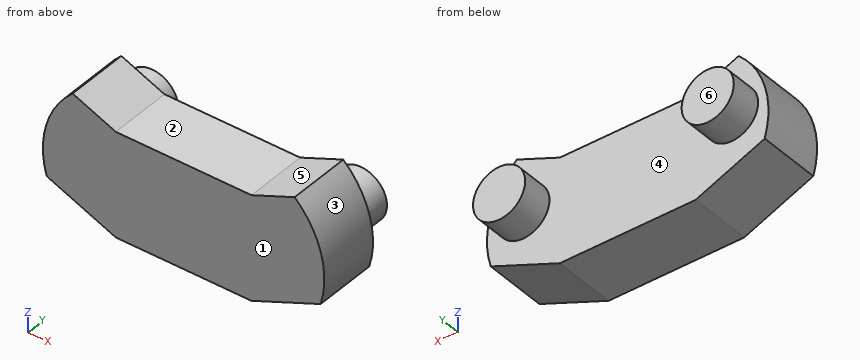
```python
from build123d import *

# Parameters (mm, degrees)
SKETCH2_W           = 32.5
SKETCH2_H           = 50
BOSS_EXTRUDE1_DEPTH = 30
FILLET1_R           = 3
SKETCH3_R           = 12.5
BOSS_EXTRUDE2_DEPTH = 45
CUT_EXTRUDE1_DEPTH  = 92.572762002


with BuildPart() as part:
    # Sketch2 → Boss-Extrude1 (new body)
    with BuildSketch(Plane(origin=(0, 0, 0), x_dir=(1, 0, 0), z_dir=(0, 1, 0))):
        with BuildLine():
            Line((-33.026431533, 15.07807147), (-21.486968519, 36.349341511))
            Line((-21.486968519, 36.349341511), (-56.486968519, 21.832088794))
            Line((-56.486968519, 21.832088794), (-47.76505884, 12.989879738))
            ThreePointArc((-47.76505884, 12.989879738), (-40.740475826, 16.467112533), (-33.026431533, 15.07807147))
        make_face()
        with BuildLine():
            Line((-47.76505884, 12.989879738), (-56.486968519, 21.832088794))
            Line((-56.486968519, 21.832088794), (-56.486968519, -28.167911206))
            Line((-56.486968519, -28.167911206), (-44.947505506, -6.896641164))
            ThreePointArc((-44.947505506, -6.896641164), (-51.3633659, 2.337207846), (-47.76505884, 12.989879738))
        make_face()
        with BuildLine():
            Line((-56.486968519, -28.167911206), (-21.486968519, -13.650658489))
            Line((-21.486968519, -13.650658489), (-30.208878198, -4.808449432))
            ThreePointArc((-30.208878198, -4.808449432), (-37.233461212, -8.285682228), (-44.947505506, -6.896641164))
            Line((-44.947505506, -6.896641164), (-56.486968519, -28.167911206))
        make_face()
        with BuildLine():
            Line((-21.486968519, -13.650658489), (-21.486968519, 36.349341511))
            Line((-21.486968519, 36.349341511), (-33.026431533, 15.07807147))
            ThreePointArc((-33.026431533, 15.07807147), (-28.245536763, 10.483808601), (-26.486968519, 4.090715153))
            ThreePointArc((-26.486968519, 4.090715153), (-27.454923405, -0.732347722), (-30.208878198, -4.808449432))
            Line((-30.208878198, -4.808449432), (-21.486968519, -13.650658489))
        make_face()
        with Locations((-5.236968519, 11.349341511)):
            Rectangle(SKETCH2_W, SKETCH2_H)
        with BuildLine():
            Line((55.052494494, 15.07807147), (43.513031481, 36.349341511))
            Line((43.513031481, 36.349341511), (43.513031481, -13.650658489))
            Line((43.513031481, -13.650658489), (52.23494116, -4.808449432))
            ThreePointArc((52.23494116, -4.808449432), (48.6366341, 5.84422246), (55.052494494, 15.07807147))
        make_face()
        with BuildLine():
            Line((78.513031481, 21.832088794), (43.513031481, 36.349341511))
            Line((43.513031481, 36.349341511), (55.052494494, 15.07807147))
            ThreePointArc((55.052494494, 15.07807147), (62.766538788, 16.467112533), (69.791121802, 12.989879738))
            Line((69.791121802, 12.989879738), (78.513031481, 21.832088794))
        make_face()
        with BuildLine():
            Line((78.513031481, -28.167911206), (78.513031481, 21.832088794))
            Line((78.513031481, 21.832088794), (69.791121802, 12.989879738))
            ThreePointArc((69.791121802, 12.989879738), (72.545076595, 8.913778028), (73.513031481, 4.090715153))
            ThreePointArc((73.513031481, 4.090715153), (71.754463237, -2.302378295), (66.973568467, -6.896641164))
            Line((66.973568467, -6.896641164), (78.513031481, -28.167911206))
        make_face()
        with BuildLine():
            Line((52.23494116, -4.808449432), (43.513031481, -13.650658489))
            Line((43.513031481, -13.650658489), (78.513031481, -28.167911206))
            Line((78.513031481, -28.167911206), (66.973568467, -6.896641164))
            ThreePointArc((66.973568467, -6.896641164), (59.259524174, -8.285682228), (52.23494116, -4.808449432))
        make_face()
        with Locations((27.263031481, 11.349341511)):
            Rectangle(SKETCH2_W, SKETCH2_H)
    extrude(amount=BOSS_EXTRUDE1_DEPTH)

    # Fillet1
    fillet1_edges = [part.edges().sort_by_distance(p)[0] for p in [
        (-56.486968519, 15, 28.167911206),
        (-56.486968519, 15, -21.832088794),
        (78.513031481, 15, -21.832088794),
        (78.513031481, 15, 28.167911206),
    ]]
    fillet(fillet1_edges, radius=FILLET1_R)

    # Sketch3 → Boss-Extrude2 (add)
    with BuildSketch(Plane(origin=(0, 0, 0), x_dir=(-1, 0, 0), z_dir=(0, -1, 0))):
        with Locations(Location((38.986968519, 4.090715153, 0), (0, 0, 90))):
            Circle(SKETCH3_R)
        with Locations(Location((-61.013031481, 4.090715153, 0), (0, 0, 90))):
            Circle(SKETCH3_R)
    extrude(amount=-BOSS_EXTRUDE2_DEPTH)

    # Sketch4 → Cut-Extrude1 (cut, through all)
    with BuildSketch(Plane(origin=(0, 30, 0), x_dir=(1, 0, 0), z_dir=(0, 1, 0))):
        with BuildLine():
            ThreePointArc((-56.486968519, -23.675749532), (-55.153077724, -26.17056017), (-52.337581774, -26.446834177))
            Line((-52.337581774, -26.446834177), (-42.18410533, -22.235388934))
            ThreePointArc((-42.18410533, -22.235388934), (-54.833584995, -1.601840339), (-54.636355265, 22.59968366))
            ThreePointArc((-54.636355265, 22.59968366), (-55.981779157, 21.494708219), (-56.486968519, 19.828599015))
            Line((-56.486968519, 19.828599015), (-56.486968519, -23.675749532))
        make_face()
        with BuildLine():
            Line((64.210168291, -22.235388934), (74.363644735, -26.446834177))
            ThreePointArc((74.363644735, -26.446834177), (77.179140685, -26.17056017), (78.513031481, -23.675749532))
            Line((78.513031481, -23.675749532), (78.513031481, 19.828599015))
            ThreePointArc((78.513031481, 19.828599015), (78.007842119, 21.494708219), (76.662418226, 22.59968366))
            ThreePointArc((76.662418226, 22.59968366), (76.859647957, -1.601840339), (64.210168291, -22.235388934))
        make_face()
    extrude(amount=-CUT_EXTRUDE1_DEPTH, mode=Mode.SUBTRACT)


solid = part.part
```
Geometry: final body of the model. Coordinates: model frame, mm. Face numbers are marked on the shaded views. A direction names the side the tool comes from. Give positions to 0.01 mm unless a question says otherwise; leave off trailing zeros. Write each loop counter-clockwise with the first axis right and the second up, starting at its lowest first coordinate (ties: lowest second). Pieces come first, ordered by that corner, then holes.
1. Line query: probe 1 along Z at (x, y) = (-12.5, 7.5); probe 2 along Y at (x, z) = (64, 14); probe 3 along X at (y, z) = (18, 16). Output: solid intervals per line, ascending.
2. Draft query along X for the marked faces 1, 2 and 3. Return one class per face: released by +X, released by -X, zero draft, split by the parting line, or undercut.
3. Section query C-C, the plane z = 2. Return loops of the section in (x, y), then the cut area to 3 significant figures.
4. Section query D-D, the plane x = -1.5. Return loops of the section in (y, z).
5. Pin query (flat end, axial travel): P1, Ø4, axis at y = 27, z = -21.5, coming from the +X side; P2, Ø4, axis at y = 18.5, z = 2.5, coming from the +X side; P3, Ø4, axis at x = 5.5, y = 29, coming from the +Z side. Return the tip coordinate at first contact, or that it passes through.
6. Reachability of the marked faces 4, 5 and 6 from +Z, -Z, +X, -X, +Y, -Y: full face, straight path, thin tool, end or side. Return the list, or none.
7. Section query A-A, the plane z = 17. Return loops of the section in (x, y), then the cut area to 3 significant figures.
8. Section query B-B, the plane y = 11. Return loops of the section in (x, z).
Computed:
1. probe 1: z = -36.35 to 13.65
1. probe 2: y = 0 to 30
1. probe 3: x = -47.8 to -27.15, 49.18 to 69.83
2. face 1: zero draft
2. face 2: undercut
2. face 3: released by +X
3. outline: (-54.72, 0) - (76.75, 0) - (76.75, 30) - (71.93, 30) - (71.93, 45) - (50.1, 45) - (50.1, 30) - (-28.07, 30) - (-28.07, 45) - (-49.9, 45) - (-49.9, 30) - (-54.72, 30) - close
3. area: 4,600 mm2
4. outline: (0, -36.35) - (30, -36.35) - (30, 13.65) - (0, 13.65) - close
5. P1: stops at x = 77.46
5. P2: stops at x = 77.15
5. P3: stops at z = 13.65
6. face 4: +Y
6. face 5: +Z, +Y, -Y
6. face 6: +Z, -Z, +X, -X, +Y
7. outline: (-47.04, 0) - (-29.56, 0) - (-29.56, 30) - (-47.04, 30) - close; (51.59, 0) - (69.06, 0) - (69.06, 30) - (51.59, 30) - close
7. area: 1,050 mm2
8. outline: (-54.64, -22.6) - (-21.49, -36.35) - (43.51, -36.35) - (76.66, -22.6) arc R43.93 ccw to (64.21, 22.24) - (43.51, 13.65) - (-21.49, 13.65) - (-42.18, 22.24) arc R43.93 ccw to start
